Geometry check sheet. Reference: the model listing, model coordinates, mm. Round coordinates to 2 decimals unless told otherwise and drop trailing zeros. Write each loop counter-clockwise with the first axis right and the second up, starting at its lowest first coordinate (ties: lowest second). Pieces come first, ordered by that corner, then holes. Notation, with made-up numbers: (29, 21.5) -> (33, 21.5) arc R21 ccw to (33, 40.5) -> close; hole circle Ø5 at (-18, 22.25). An arc over 180 degrees is marked (long way). Return JSON: item names as keys, results as strings. Group by question number.
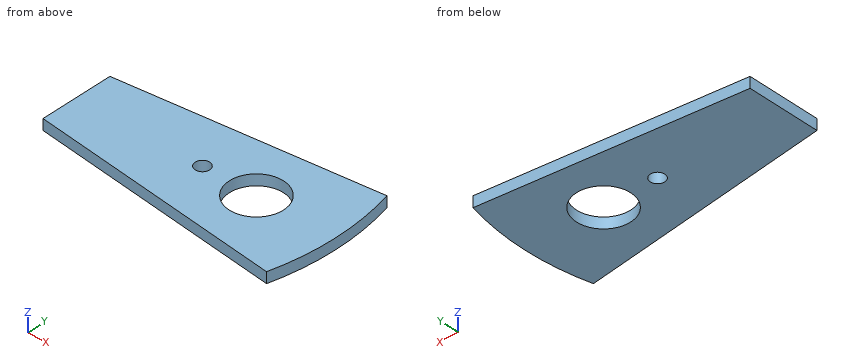
from build123d import *

# Parameters (mm, degrees)
F0_R     = 2
F0_R_2   = 7.5
F1_DEPTH = 3


with BuildPart() as f1:
    # F0 (on Top) → F1 (new body)
    with BuildSketch(Plane.XY):
        with BuildLine():
            ThreePointArc((34.541355, -18), (36.83314, 0), (34.541355, 18))
            Line((34.541355, 18), (-35, 10))
            Line((-35, 10), (-35, -10))
            Line((-35, -10), (34.541355, -18))
        make_face()
        Circle(F0_R, mode=Mode.SUBTRACT)
        with Locations((15, 0)):
            Circle(F0_R_2, mode=Mode.SUBTRACT)
    extrude(amount=F1_DEPTH)


solid = f1.part
1) Sectioned sample at C-C on x = 19. Enter the section's corners in (y, z).
2) Sectioned sample at B-B on z = 1.45. Enter the section's corners in (x, y).
3) Material ranges on probe 1 along X at (y, z) = (-6, 2.05); probe 2 along X at (y, z) = (3.5, 2.1); probe 3 along Y at (x, z) = (17, 2.05), recorded low to high. Write a range as [from, to].
4) Sectioned sample at D-D on y = -6. Enter the section's corners in (x, z).
5) Sectioned sample at A-A on y = 0. Enter the section's corners in (x, z).
6) Go/stop test with flat-tipped pins: P1, Ø1, axis at x = 7.5, y = -1.5, coming from the -Z side; P2, Ø1, axis at x = 10, z = 2, coming from the +Y side. Record where each tip stops, or that it passes through.
Evaluation:
{
 "1": {"outline": "(-16.21, 0) -> (-6.34, 0) -> (-6.34, 3) -> (-16.21, 3) -> close; (6.34, 0) -> (16.21, 0) -> (16.21, 3) -> (6.34, 3) -> close"},
 "2": {"outline": "(-35, -10) -> (34.54, -18) arc R71.83 ccw to (34.54, 18) -> (-35, 10) -> close; hole circle Ø4 at (0, 0); hole circle Ø15 at (15, 0)"},
 "3": {"probe 1": "x = [-35, 10.5], [19.5, 36.58]", "probe 2": "x = [-35, 8.37], [21.63, 36.75]", "probe 3": "y = [-15.98, -7.23], [7.23, 15.98]"},
 "4": {"outline": "(-35, 0) -> (10.5, 0) -> (10.5, 3) -> (-35, 3) -> close; (19.5, 0) -> (36.58, 0) -> (36.58, 3) -> (19.5, 3) -> close"},
 "5": {"outline": "(-35, 0) -> (-2, 0) -> (-2, 3) -> (-35, 3) -> close; (2, 0) -> (7.5, 0) -> (7.5, 3) -> (2, 3) -> close; (22.5, 0) -> (36.83, 0) -> (36.83, 3) -> (22.5, 3) -> close"},
 "6": {"P1": "stops at z = 0", "P2": "stops at y = 15.23"}
}
